Can you work these out from the drawing? Everything is in mm from the part's minimum corner. A direction names the side the tool comes from. Round coordinates to 2 decimals unless told otherwise and drop trailing zeros. Loops run counter-clockwise (first coordinate to the right, second up) from the corner with the lowest first, then second, coordinate; pieces in that order, holes last. Notation, with made-up numbers: (77, 53) -> (87, 53) arc R29 ccw to (87, 79) -> close; hole circle Ø3 at (80, 87). An arc over 180 degrees is marked (long way). Use CSV: the item, a comma, the result in double quotes. Start each with the question number.
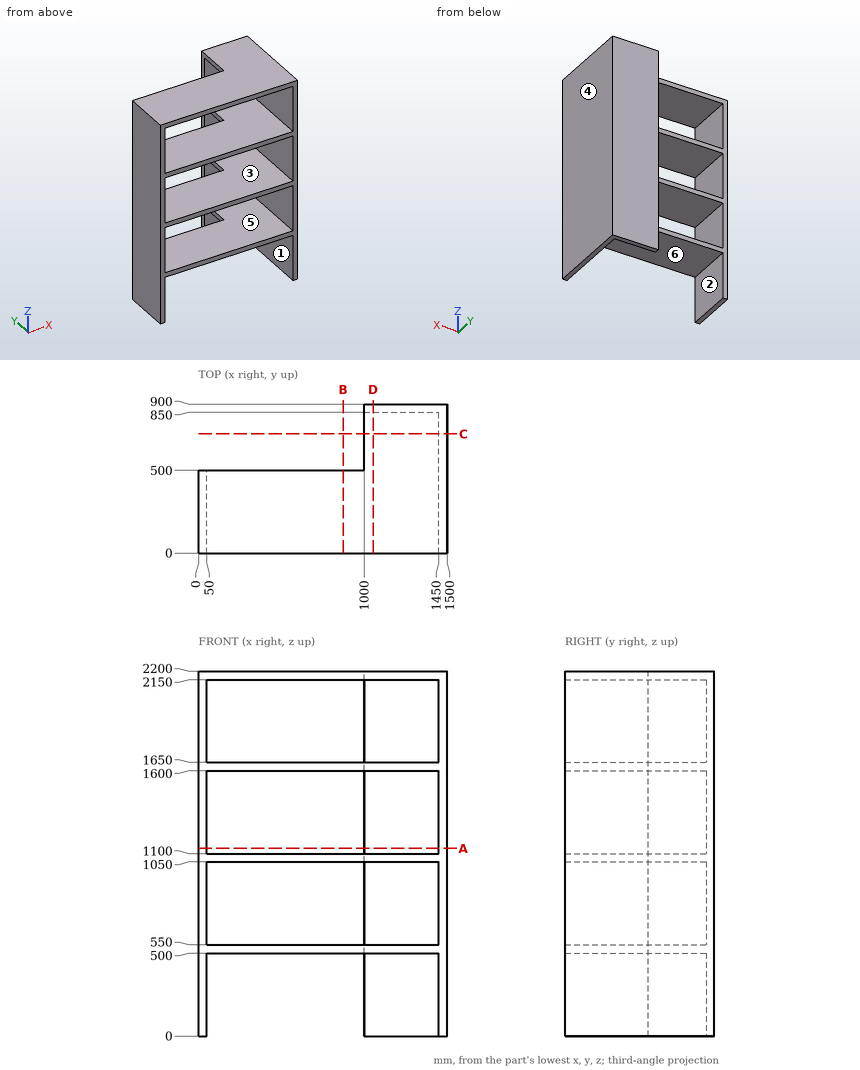
1. Will these pins go through, and if not, where does the flat tip stop? pin 1 (12 mm diameter, centred on x = 1013, z = 375.5, fed in from -Y); pin 2 (3 mm diameter, centred on y = 101.5, z = 931.5, fed in from -X).
2. Suppose I cut it at D-D (x = 1053). List the corners of the cut face in (y, z) for me.
3. Suppose I cut it at C-C (y = 720.5). List the corners of the cut face in (x, z) for me.
4. We'd pull the mould along Z, two halves only. Please class the marked faces 4, 5 and 6: pulls with the +Z half, pulls with the -Z half, needs draft (parallel to the pull), parting line crosses it, or undercut.
5. Suppose I cut it at B-B (x = 872.5). List the corners of the cut face in (y, z) for me, then the cut area to 3 significant figures.
6. Suppose I cut it at A-A (z = 1132). List the corners of the cut face in (x, y) for me.
7. If I drill on L1, parallel to Z at x = 1370.5, y = 802.5; L2, parallel to X at y = 75, z = 316.5; L3, parallel to Y at x = 1034, z = 2104, over which ranges is the centre line in solid material (lowest first)?
8. For the marked faces 1, 2 and 3, which set-ups out of +Z, -Z, +X, -X, +Y, -Y let a thin tool reach every point of the face, with its end or its side?
Geometry check:
1,pin 1,"stops at y = 850"
1,pin 2,"stops at x = 0"
2,outline,"(0, 500) -> (850, 500) -> (850, 0) -> (900, 0) -> (900, 2200) -> (0, 2200) -> (0, 2150) -> (850, 2150) -> (850, 1650) -> (0, 1650) -> (0, 1600) -> (850, 1600) -> (850, 1100) -> (0, 1100) -> (0, 1050) -> (850, 1050) -> (850, 550) -> (0, 550) -> close"
3,outline,"(1000, 500) -> (1450, 500) -> (1450, 0) -> (1500, 0) -> (1500, 2200) -> (1000, 2200) -> (1000, 2150) -> (1450, 2150) -> (1450, 1650) -> (1000, 1650) -> (1000, 1600) -> (1450, 1600) -> (1450, 1100) -> (1000, 1100) -> (1000, 1050) -> (1450, 1050) -> (1450, 550) -> (1000, 550) -> close"
4,face 4,"needs draft"
4,face 5,"undercut"
4,face 6,"pulls with the -Z half"
5,outline,"(0, 500) -> (500, 500) -> (500, 550) -> (0, 550) -> close; (0, 1050) -> (500, 1050) -> (500, 1100) -> (0, 1100) -> close; (0, 1600) -> (500, 1600) -> (500, 1650) -> (0, 1650) -> close; (0, 2150) -> (500, 2150) -> (500, 2200) -> (0, 2200) -> close"
5,area,"100,000 mm²"
6,outline,"(0, 0) -> (50, 0) -> (50, 500) -> (0, 500) -> close; (1000, 850) -> (1450, 850) -> (1450, 0) -> (1500, 0) -> (1500, 900) -> (1000, 900) -> close"
7,L1,"z = 500 to 550, 1050 to 1100, 1600 to 1650, 2150 to 2200"
7,L2,"x = 0 to 50, 1450 to 1500"
7,L3,"y = 850 to 900"
8,face 1,"-Z, -Y"
8,face 2,"-Z, +Y, -Y"
8,face 3,"-Y"
